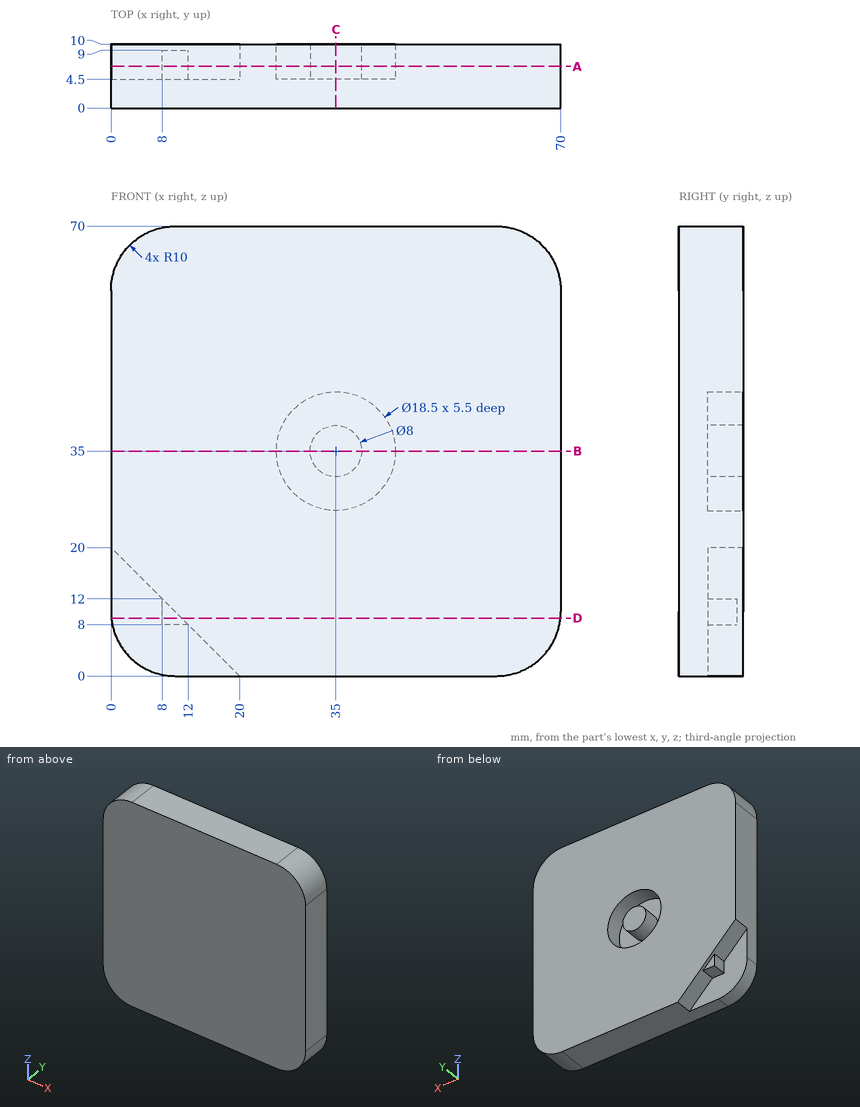
Geometry: see drawing. Coordinates: mm, zero at the bounding-box minimum. Coordinates: 2 decimals unless noted, no trailing zeros. Write each loop counter-clockwise with the first axis right and the second up, starting at its lowest first coordinate (ties: lowest second). Pieces come first, ordered by that corner, then holes.
1) Pin query (flat end, axial travel): pin 1 Ø8 at (x, z) = (32.5, 28) entering from -Y; pin 2 Ø1.2 at (x, y) = (10, 6.5) entering from -Z; pin 3 Ø1.2 at (y, z) = (8, 11) entering from -X. Return the tip coordinate at first contact, or that it passes through.
2) Section C-C on x = 35. Output: boundary loops of the cut face in (y, z), and give its area (3 significant figures).
3) Section B-B on z = 35. Output: boundary loops of the cut face in (x, y).
4) Section D-D on z = 9. Output: boundary loops of the cut face in (x, y).
5) Material intervals for line 1 along Z through (x, y) = (35, 6.9); line 2 along X through (y, z) = (5.25, 36), sorted ascending.
6) Section A-A on y = 6.5. Output: boundary loops of the cut face in (x, z).
Check result:
1. pin 1: stops at y = 0
1. pin 2: stops at z = 8
1. pin 3: stops at x = 8
2. outline: (0, 0) - (10, 0) - (10, 25.75) - (4.5, 25.75) - (4.5, 31) - (10, 31) - (10, 39) - (4.5, 39) - (4.5, 44.25) - (10, 44.25) - (10, 70) - (0, 70) - close
2. area: 642 mm2
3. outline: (0, 0) - (70, 0) - (70, 10) - (44.25, 10) - (44.25, 4.5) - (39, 4.5) - (39, 10) - (31, 10) - (31, 4.5) - (25.75, 4.5) - (25.75, 10) - (0, 10) - close
4. outline: (0.05, 0) - (69.95, 0) - (69.95, 10) - (11, 10) - (11, 9) - (8, 9) - (8, 4.5) - (0.05, 4.5) - close
5. line 1: z = 0 to 25.75, 31 to 39, 44.25 to 70
5. line 2: x = 0 to 25.8, 31.13 to 38.87, 44.2 to 70
6. outline: (0, 20) - (8, 12) - (8, 8) - (12, 8) - (20, 0) - (60, 0) arc R10 ccw to (70, 10) - (70, 60) arc R10 ccw to (60, 70) - (10, 70) arc R10 ccw to (0, 60) - close; circle Ø8 at (35, 35); hole circle Ø18.5 at (35, 35)
